from build123d import *

# Parameters (mm, degrees)
SM_BASE_FLANGE_1_DEPTH      = 2
SM_EDGE_FLANGE_1_DEPTH      = 5
SM_EDGE_FLANGE_1_BEND_DEPTH = 5
SKETCH_16_W                 = 1
SKETCH_16_H                 = 1
CUT_EXTRUDE_3_DEPTH         = 0.3


# Sheet-metal steps are written as plain solids
with BuildPart() as part:
    # Эскиз5 → Базовая кромка1 (new body)
    with BuildSketch(Plane.XY):
        with BuildLine():
            Line((-8.670207128, -3.533537369), (-8.670207128, -0.625462256))
            ThreePointArc((-8.670207128, -0.625462256), (-8.643827777, -0.557786558), (-8.578607126, -0.52581568))
            Line((-8.578607126, -0.52581568), (2.29091619, 0.390462415))
            Line((2.29091619, 0.390462415), (2.274116194, 0.589755566))
            Line((2.274116194, 0.589755566), (-8.595407122, -0.326522529))
            ThreePointArc((-8.595407122, -0.326522529), (-8.791069074, -0.422435162), (-8.870207128, -0.625462256))
            Line((-8.870207128, -0.625462256), (-8.870207128, -3.533537369))
            Line((-8.870207128, -3.533537369), (-8.670207128, -3.533537369))
        make_face()
    extrude(amount=SM_BASE_FLANGE_1_DEPTH)

    # Ребро-кромка1 section (across the edge) → Ребро-кромка1 (add)
    with BuildSketch(Plane(origin=(-2.708212587, 0.169755664, 2.1), x_dir=(0, 0, -1), z_dir=(0.9964657562113037, 0.08399998034663243, 0))):
        with BuildLine():
            Line((-0.2, 0.1), (-0.2, 0.3))
            Line((-0.2, 0.3), (0, 0.3))
            Line((0, 0.3), (0, 0.1))
            ThreePointArc((0, 0.1), (0.029289322, 0.029289322), (0.1, 0))
            Line((0.1, 0), (0.1, -0.2))
            ThreePointArc((0.1, -0.2), (-0.112132034, -0.112132034), (-0.2, 0.1))
        make_face()
    extrude(amount=SM_EDGE_FLANGE_1_DEPTH)

    # Ребро-кромка1 section 2 (across the edge) → Ребро-кромка1 bend (add)
    with BuildSketch(Plane(origin=(2.274116194, 0.589755566, -0.1), x_dir=(0, 0, 1), z_dir=(-0.9964657562113037, -0.08399998034663243, 0))):
        with BuildLine():
            Line((-0.2, 0.1), (-0.2, 0.3))
            Line((-0.2, 0.3), (0, 0.3))
            Line((0, 0.3), (0, 0.1))
            ThreePointArc((0, 0.1), (0.029289322, 0.029289322), (0.1, 0))
            Line((0.1, 0), (0.1, -0.2))
            ThreePointArc((0.1, -0.2), (-0.112132034, -0.112132034), (-0.2, 0.1))
        make_face()
    extrude(amount=SM_EDGE_FLANGE_1_BEND_DEPTH)

    # Эскиз16 → Вырез-Вытянуть3 (cut)
    with BuildSketch(Plane(origin=(-0.033318215, 0.395243668, 0), x_dir=(0.9964657562113037, 0.08399998034663245, 0), z_dir=(-0.08399998034663245, 0.9964657562113038, 0))):
        with Locations((0.315618369, -1)):
            Rectangle(SKETCH_16_W, SKETCH_16_H)
    extrude(amount=-CUT_EXTRUDE_3_DEPTH, mode=Mode.SUBTRACT)


solid = part.part
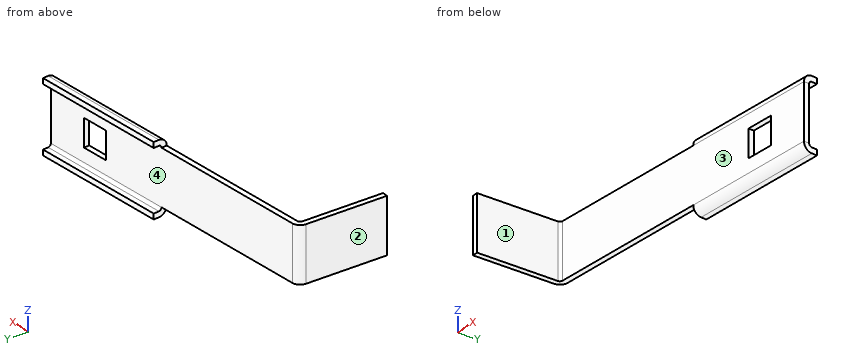
Work out the finished part from the listing and answer in its coordinate system (mm). Face numbers are marked on the shaded views. A direction names the side the tool comes from. Round coordinates to 2 decimals unless told otherwise and drop trailing zeros. Loops run counter-clockwise (first coordinate to the right, second up) from the corner with the lowest first, then second, coordinate; pieces in that order, holes last. Notation, with made-up numbers: (-24, 42) -> (0, 42) arc R20 cw to (0, 78) -> close; hole circle Ø5 at (-37, 33). An arc over 180 degrees is marked (long way). Use one line per item in the form item = value.
(1) For a pull along Z with two mould halves and no side action, classify the marked faces 3 and 4 as released by +Z, released by -Z, zero draft, split by the parting line, or undercut.
Answer list:
face_3 = zero draft
face_4 = undercut
(2) Find section D-D on x = -3. Give the vertices of the cut face in (y, z), then the cut area to 3 significant figures.
Answer list:
outline = (-0.06, 0) -> (0.15, 0) -> (0.15, 2) -> (-0.06, 2) -> close
area = 0.401 mm2
(3) Straight lines are drawn through the part: line 1 (X direction, y = -1.65, z = 1.05); line 2 (Y direction, x = -7.75, z = 0.5); line 3 (Y direction, x = -2.5, z = 0.5). For each, find the intervals that lie inside material, in ascending order.
Answer list:
line_1 = -8.87 to -8.67
line_2 = -0.46 to -0.26
line_3 = -0.01 to 0.19
(4) A tool of negligible diameter and unlimited length cuts with its end or side. For the marked faces 1 and 2, from which of +Z, -Z, +X, -X, +Y, -Y can it reach the whole face along a straight path? Write none if from no direction.
Answer list:
face_1 = +Z, -Z, +X, -Y
face_2 = +Z, -Z, -X, +Y, -Y
(5) Find section A-A on z = 0.8. Give the vertices of the cut face in (x, y), then the cut area to 3 significant figures.
Answer list:
outline = (-8.87, -3.53) -> (-8.67, -3.53) -> (-8.67, -0.63) arc R0.1 cw to (-8.58, -0.53) -> (-0.2, 0.18) -> (-0.22, 0.38) -> (-8.6, -0.33) arc R0.3 ccw to (-8.87, -0.63) -> close; (0.78, 0.46) -> (0.8, 0.26) -> (2.29, 0.39) -> (2.27, 0.59) -> close
area = 2.62 mm2
(6) Find section B-B on z = 1.6. Give the vertices of the cut face in (x, y), then the cut area to 3 significant figures.
Answer list:
outline = (-8.87, -3.53) -> (-8.67, -3.53) -> (-8.67, -0.63) arc R0.1 cw to (-8.58, -0.53) -> (2.29, 0.39) -> (2.27, 0.59) -> (-8.6, -0.33) arc R0.3 ccw to (-8.87, -0.63) -> close
area = 2.82 mm2
(7) Find section C-C on y = -2.4. Give the vertices of the cut face in (x, z), then the cut area to 3 significant figures.
Answer list:
outline = (-8.87, 0) -> (-8.67, 0) -> (-8.67, 2) -> (-8.87, 2) -> close
area = 0.400 mm2
(8) Flat-ended cylindrical pins translate along their axes: P1, Ø1.5, axis at x = -7.5, z = 1, coming from the +Y side; P2, Ø1.9, axis at x = -7, y = -1, coming from the +Z side; P3, Ø1, axis at y = -1.5, z = 0.5, coming from the +X side. Find the tip coordinate at first contact, or state that the pin passes through.
Answer list:
P1 = -0.17
P2 = 2
P3 = -8.67
